```python
from build123d import *

# Parameters (mm, degrees)
SKETCH1_R           = 4.845
SKETCH1_R_2         = 1.5
BOSS_EXTRUDE1_DEPTH = 8.89
SKETCH2_R           = 1.5
BOSS_EXTRUDE2_DEPTH = 7.5
SKETCH3_R           = 1.95
BOSS_EXTRUDE3_DEPTH = 6.5


with BuildPart() as part:
    # Sketch1 → Boss-Extrude1 (new body)
    with BuildSketch(Plane.XY):
        with Locations(Location((0, 0, 0), (0, 0, 180))):
            Circle(SKETCH1_R)
        with Locations(Location((0, 0, 0), (0, 0, 180))):
            Circle(SKETCH1_R_2, mode=Mode.SUBTRACT)
    extrude(amount=BOSS_EXTRUDE1_DEPTH)

    # Sketch2 → Boss-Extrude2 (add)
    with BuildSketch(Plane.XY.offset(8.89)):
        with BuildLine():
            Line((-2.236067977, 2), (2.236067977, 2))
            ThreePointArc((2.236067977, 2), (3, 0), (2.236067977, -2))
            Line((2.236067977, -2), (-2.236067977, -2))
            ThreePointArc((-2.236067977, -2), (-3, 0), (-2.236067977, 2))
        make_face()
        with Locations(Location((0, 0, 0), (0, 0, 180))):
            Circle(SKETCH2_R, mode=Mode.SUBTRACT)
    extrude(amount=BOSS_EXTRUDE2_DEPTH)

    # Sketch3 → Boss-Extrude3 (add)
    with BuildSketch(Plane.XY.offset(16.39)):
        with Locations(Location((0, 0, 0), (0, 0, 180))):
            Circle(SKETCH3_R)
    extrude(amount=BOSS_EXTRUDE3_DEPTH)


solid = part.part
```
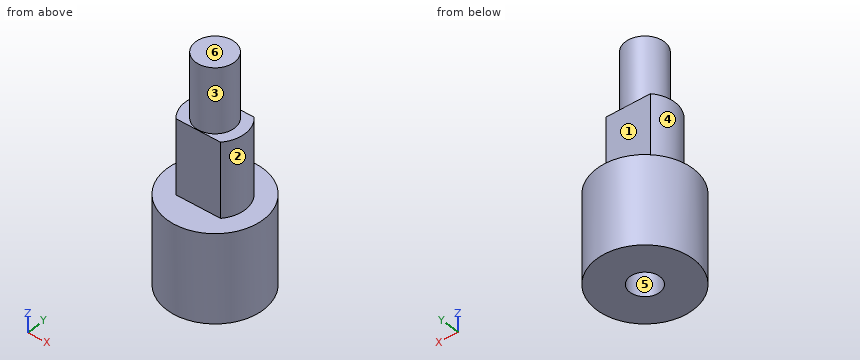
Part model, mm, in its own coordinate system. Face numbers are marked on the shaded views. A direction names the side the tool comes from. Round coordinates to 2 decimals unless told otherwise and drop trailing zeros. Loops run counter-clockwise (first coordinate to the right, second up) from the corner with the lowest first, then second, coordinate; pieces in that order, holes last. Notation, with made-up numbers: (42, -23.75) -> (91, -23.75) arc R26 cw to (91, -8.75) -> close; hole circle Ø11 at (-1, -4). An arc over 180 degrees is marked (long way). Use a Markdown table: item, result.
1) Cut at D-D, the plane z = 19.5. List the corners of the cut face in (x, y).
The answers:
| item | result |
|---|---|
| outline | circle Ø3.9 at (0, 0) |
2) Cut at B-B, the plane y = 0. List the corners of the cut face in (x, z) (3 decimals), and give its area (3 significant figures).
The answers:
| item | result |
|---|---|
| outline | (-4.845, 0) -> (-1.5, 0) -> (-1.5, 16.39) -> (1.5, 16.39) -> (1.5, 0) -> (4.845, 0) -> (4.845, 8.89) -> (3, 8.89) -> (3, 16.39) -> (1.95, 16.39) -> (1.95, 22.89) -> (-1.95, 22.89) -> (-1.95, 16.39) -> (-3, 16.39) -> (-3, 8.89) -> (-4.845, 8.89) -> close |
| area | 107 mm2 |
3) Cut at C-C, the plane x = 0. List the corners of the cut face in (y, z) (3 decimals).
The answers:
| item | result |
|---|---|
| outline | (-4.845, 0) -> (-1.5, 0) -> (-1.5, 16.39) -> (1.5, 16.39) -> (1.5, 0) -> (4.845, 0) -> (4.845, 8.89) -> (2, 8.89) -> (2, 16.39) -> (1.95, 16.39) -> (1.95, 22.89) -> (-1.95, 22.89) -> (-1.95, 16.39) -> (-2, 16.39) -> (-2, 8.89) -> (-4.845, 8.89) -> close |
4) Drop flat-ended pins along their axis: pin 1 Ø3.5 at (x, z) = (1, 13.5) entering from +Y; pin 2 Ø1.3 at (x, z) = (0, 11.5) entering from -Y; pin 3 Ø5 at (x, z) = (-3.5, 4) entering from -Y. Give the stop position or say it passes through.
The answers:
| item | result |
|---|---|
| pin 1 | stops at y = 2 |
| pin 2 | stops at y = -2 |
| pin 3 | stops at y = -4.74 |
5) Probe line 1 (Y direction, x = 0, z = 13); line 2 (Y direction, x = 0, z = 6.5) (3 decimals); line 3 (Z direction, x = 2, y = 4.25). List the from-to ranges inside material, lowest first. Write a range as [from, to].
The answers:
| item | result |
|---|---|
| line 1 | y = [-2, -1.5], [1.5, 2] |
| line 2 | y = [-4.845, -1.5], [1.5, 4.845] |
| line 3 | z = [0, 8.89] |
6) Cut at A-A, the plane z = 9.25. List the corners of the cut face in (x, y), and give its area (3 significant figures).
The answers:
| item | result |
|---|---|
| outline | (-2.24, -2) -> (2.24, -2) arc R3 ccw to (2.24, 2) -> (-2.24, 2) arc R3 ccw to start; hole circle Ø3 at (0, 0) |
| area | 15.0 mm2 |
7) Pull direction Y, two halves, no side cores. Call the marked faces 4, 5 and 6: pulls with the +Y half, pulls with the -Y half, needs draft (parallel to the pull), parting line crosses it, or undercut.
The answers:
| item | result |
|---|---|
| face 4 | parting line crosses it |
| face 5 | undercut |
| face 6 | needs draft |
8) Tool access for the marked faces 1, 2 and 3: list every direction of +Z, -Z, +X, -X, +Y, -Y with a clear straight run to the whole face (end or side of a thin tool).
The answers:
| item | result |
|---|---|
| face 1 | +Z, +X, -X, +Y |
| face 2 | +Z, +X |
| face 3 | +Z |
